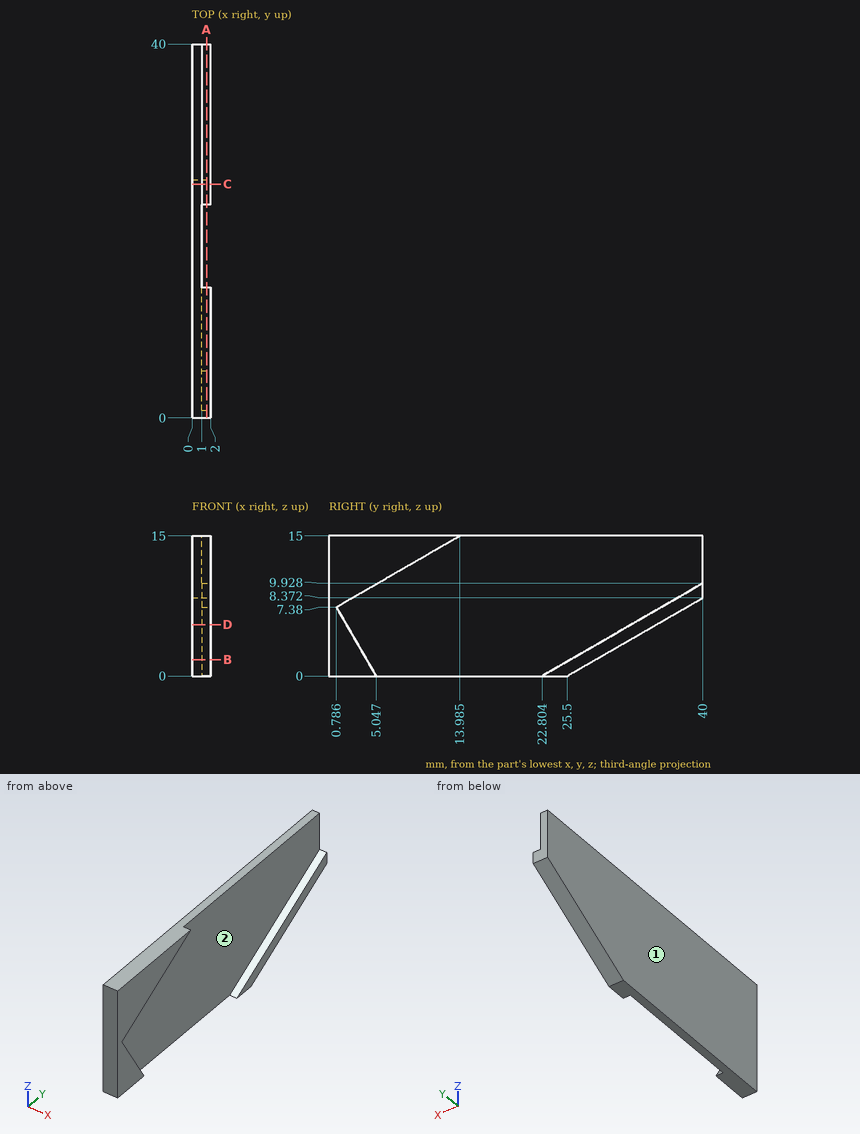
Study the drawing (mm; zero at the part's minimum x, y, z) and answer. Round coordinates to 2 decimals unless told otherwise and drop trailing zeros. Write each loop counter-clockwise with the first axis right and the second up, starting at its lowest first coordinate (ties: lowest second). Pieces come first, ordered by that corner, then holes. Notation, with made-up numbers: (7, 54.25) -> (59, 54.25) arc R26 ccw to (59, 83.25) -> close; hole circle Ø6 at (12.25, 72.5). An arc over 180 degrees is marked (long way). Write item = value, one per line.
1) Straight lines are drawn through the part: line 1 along Y through (x, z) = (1.85, 7.75) (1 decimal); line 2 along Z through (x, y) = (1.75, 4) (1 decimal); line 3 along Y through (x, z) = (1.4, 3.25) (1 decimal). For each, find the intervals that lie inside material, in ascending order. Write a range as [from, to].
Check values:
line_1 = [0, 1.4], [36.2, 38.9]
line_2 = [0, 1.8], [9.2, 15]
line_3 = [0, 3.2], [28.4, 31.1]
2) Section C-C on y = 25 is taken. Write down the section's boundary in (x, z).
Check values:
outline = (0, 0) -> (2, 0) -> (2, 1.27) -> (1, 1.27) -> (1, 15) -> (0, 15) -> close
3) Section B-B on z = 1.75 is taken. Write down the section's boundary in (x, y) (1 decimal).
Check values:
outline = (0, 0) -> (2, 0) -> (2, 4) -> (1, 4) -> (1, 25.8) -> (2, 25.8) -> (2, 28.5) -> (0, 28.5) -> close
4) For a pull along Y with two mould halves and no side action, classify the marked faces 1 and 2 as released by +Y, released by -Y, zero draft, split by the parting line, or undercut.
Check values:
face_1 = zero draft
face_2 = undercut
5) Given pin 1 (1 mm diameter, centred on x = 1, z = 10.5, fed in from -Y); pin 2 (1 mm diameter, centred on y = 28.5, z = 4, fed in from +X), each flat-ended and moving along its own axis, determine where each tip first touches the part or whether it passes through.
Check values:
pin_1 = 0
pin_2 = 1
6) Section D-D on z = 5.5 is taken. Write down the section's boundary in (x, y).
Check values:
outline = (0, 0) -> (2, 0) -> (2, 1.87) -> (1, 1.87) -> (1, 32.33) -> (2, 32.33) -> (2, 35.03) -> (0, 35.03) -> close
7) Section A-A on x = 1.55 is taken. Write down the section's boundary in (y, z) (1 decimal).
Check values:
outline = (0, 0) -> (5, 0) -> (0.8, 7.4) -> (14, 15) -> (0, 15) -> close; (22.8, 0) -> (25.5, 0) -> (40, 8.4) -> (40, 9.9) -> close
